Verification items for the finished model (mm, model axes). Round coordinates to 2 decimals unless told otherwise and drop trailing zeros. Order: outer loops, then holes, each group sorted by start corner. A loop starts at its lowest first (then second) coordinate and runs counter-clockwise, first axis right, second up. Notation, with made-up numbers: M 10.5,18.5 L 56.5,18.5 A11 cw 56.5,25.5 Z; hole C 35.25,-29.75 d8. An arc over 180 degrees is marked long. Answer as a JSON object with one key per item and string values. Group by question number.
```python
from build123d import *

# Parameters (mm, degrees)
SKETCH1_W              = 101.6
SKETCH1_H              = 76.2
SKETCH1_R              = 9.525
BOSS_EXTRUDE1_DEPTH    = 3.175
F_8_CLEARANCE_HOLE1_D  = 4.4958
CHAMFER1_SIZE          = 25.4
F_10_CLEARANCE_HOLE2_D = 5.1054
FILLET1_R              = 6.35


with BuildPart() as part:
    # Sketch1 → Boss-Extrude1 (new, symmetric)
    with BuildSketch(Plane.XY):
        with Locations((0, -12.7)):
            Rectangle(SKETCH1_W, SKETCH1_H)
        Circle(SKETCH1_R, mode=Mode.SUBTRACT)
    extrude(amount=BOSS_EXTRUDE1_DEPTH, both=True)

    # #8 Clearance Hole1 (through all)
    with Locations(Plane.XY.offset(3.175)):
        with Locations((-17.960512242, 17.960512242), (17.960512242, -17.960512242)):
            Hole(F_8_CLEARANCE_HOLE1_D / 2)

    # Chamfer1
    chamfer1_edges = [part.edges().sort_by_distance(p)[0] for p in [
        (-50.8, 25.4, 0),
        (50.8, 25.4, 0),
    ]]
    chamfer(chamfer1_edges, length=CHAMFER1_SIZE)

    # #10 Clearance Hole2 (through all)
    with Locations(Plane.XY.offset(3.175)):
        with Locations((-38.1, -38.1), (-12.7, -38.1), (12.7, -38.1), (38.1, -38.1)):
            Hole(F_10_CLEARANCE_HOLE2_D / 2)

    # Fillet1
    fillet1_edges = [part.edges().sort_by_distance(p)[0] for p in [
        (-25.4, 25.4, 0),
        (25.4, 25.4, 0),
        (50.8, 0, 0),
        (-50.8, 0, 0),
        (50.8, -50.8, 0),
        (-50.8, -50.8, 0),
    ]]
    fillet(fillet1_edges, radius=FILLET1_R)


solid = part.part
```
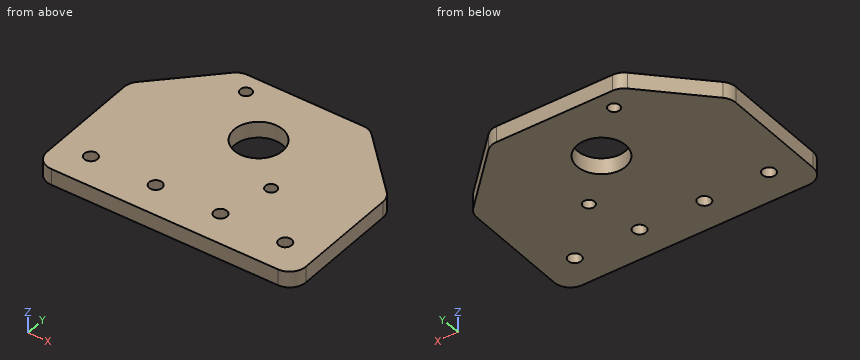
Q1. Cross-section at B-B, the plane y = 0. Record the cut outline in (x, z) (3 decimals), then the cut area to 3 significant figures.
Q2. Cross-section at C-C, the plane z = -0.5. Record the cut outline in (x, y) (3 decimals), then the cut area to 3 significant figures.
Q3. Cross-section at D-D, the plane y = 11. Record the cut outline in (x, z) (3 decimals), then the cut area to 3 significant figures.
Q4. Cross-section at A-A, the plane x = 0. Record the cut outline in (y, z) (3 decimals), then the cut area to 3 significant figures.
Q5. Thickness scan on line 1 (Y direction, x = 12.7, z = -1); line 2 (Y direction, x = 0, z = 1.5) (3 decimals); line 3 (X direction, y = -39, z = -2.25). Record the ranges inside material, lowest first. Write a range as from..to.
Q6. Gauge pin test, flat ends, axial feed: pin 1 Ø8 at (x, y) = (12.7, -38.1) entering from -Z (3 decimals); pin 2 Ø3 at (y, z) = (17, 0) entering from -X. Record the tip position at first contact, or that the pin passes through.
Conclusion:
{
 "1": {"outline": "M -50.23,-3.175 L -9.525,-3.175 L -9.525,3.175 L -50.23,3.175 Z; M 9.525,-3.175 L 50.23,-3.175 L 50.23,3.175 L 9.525,3.175 Z", "area": "517 mm2"},
 "2": {"outline": "M -50.8,-44.45 A6.35 ccw -44.45,-50.8 L 44.45,-50.8 A6.35 ccw 50.8,-44.45 L 50.8,-2.63 A6.35 ccw 48.94,1.86 L 27.26,23.54 A6.35 ccw 22.77,25.4 L -22.77,25.4 A6.35 ccw -27.26,23.54 L -48.94,1.86 A6.35 ccw -50.8,-2.63 Z; hole C -38.1,-38.1 d5.105; hole C -17.961,17.961 d4.496; hole C -12.7,-38.1 d5.105; hole C 0,0 d19.05; hole C 12.7,-38.1 d5.105; hole C 17.961,-17.961 d4.496; hole C 38.1,-38.1 d5.105", "area": "6,680 mm2"},
 "3": {"outline": "M -39.8,-3.175 L 39.8,-3.175 L 39.8,3.175 L -39.8,3.175 Z", "area": "505 mm2"},
 "4": {"outline": "M -50.8,-3.175 L -9.525,-3.175 L -9.525,3.175 L -50.8,3.175 Z; M 9.525,-3.175 L 25.4,-3.175 L 25.4,3.175 L 9.525,3.175 Z", "area": "363 mm2"},
 "5": {"line 1": "-50.8..-40.65, -35.55..25.4", "line 2": "-50.8..-9.525, 9.525..25.4", "line 3": "-50.8..-40.49, -35.71..-15.09, -10.31..10.31, 15.09..35.71, 40.49..50.8"},
 "6": {"pin 1": "z = -3.175", "pin 2": "x = -35.3"}
}
